Can you work these out from the model? Positions are in its coordinate system, mm. Face numbers are marked on the shaded views. A direction names the side the tool comes from. Give positions to 0.01 mm unless a question says otherwise; leave off trailing zeros. Order: outer loops, then holes, each group sorted by start corner. A loop starts at its lowest first (then second) coordinate and runs counter-clockwise, first axis right, second up. Notation, with made-up numbers: M 78.25,-22.75 L 135.25,-22.75 A21 cw 135.25,13.25 Z; hole C 5,-28.75 d1. An arc over 180 degrees is marked long. Use one line per item in the form item = value. Start each with the question number.
1. We'd pull the mould along Z, two halves only. Please class the marked faces 6, 7 and 8: +Z half, -Z half, draft (parallel to the pull), parting line (faces both ways), or undercut.
2. For the marked faces 1, 2, 3, 4 and 5, which set-ups out of +Z, -Z, +X, -X, +Y, -Y let a thin tool reach every point of the face, with its end or its side?
3. I want a section at D-D, the plane z = 0.5. List the corners of the cut face in (x, y) for me.
4. I want a section at C-C, the plane y = 12.5. List the corners of the cut face in (x, z) for me, and give its area (3 significant figures).
5. Will these pins go through, and if not, where does the flat tip stop? P1, Ø2.5, axis at x = -7, z = 0, coming from the -Y side; P2, Ø3, axis at y = 0.5, z = -7, coming from the -X side; P3, Ø8.5, axis at x = -4.5, y = -3, coming from the +Z side; P4, Ø1, axis at x = -8, z = -4.5, coming from the -Y side.
6. I want a section at B-B, the plane x = 5.5. List the corners of the cut face in (y, z) for me.
7. I want a section at A-A, the plane z = 4.5. List the corners of the cut face in (x, y) for me, and give its area (3 significant figures).
8. I need wall thicknesses on L1, parallel to X at y = 7, z = -5.25; L2, parallel to Z at x = 8.5, y = 3; L3, parallel to X at y = -10, z = -8. Which ranges of each line are inside material? Lowest first, please.
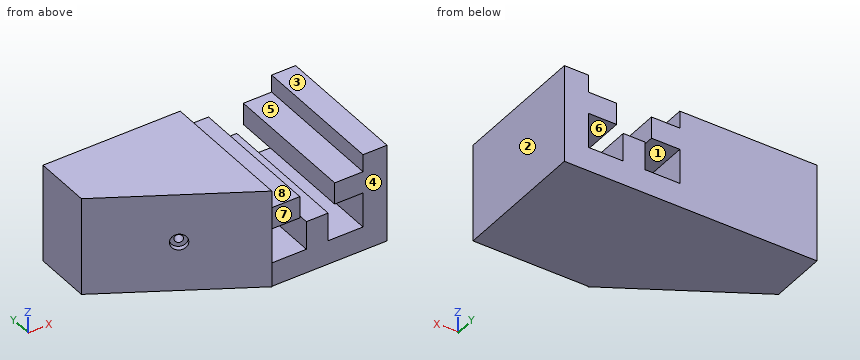
```python
from build123d import *

# Parameters (mm, degrees)
BOSS_EXTRU_1_DEPTH                               = 15
ESQUISSE1_W                                      = 21.65
ESQUISSE1_H                                      = 30
BOSS_EXTRU_2_DEPTH                               = 25
ESQUISSE3_W                                      = 30.3
ESQUISSE3_H                                      = 21.65
BOSS_EXTRU_3_DEPTH                               = 25
ENL_V_MAT_EXTRU_2_DEPTH                          = 61.834878976
ENL_V_MAT_EXTRU_2_DEPTH_BACK                     = 61.834878976
CHAMBRAGE_POUR_VIS_T_TE_RONDE_BOMB_E_D           = 1.778
CHAMBRAGE_POUR_VIS_T_TE_RONDE_BOMB_E_DEPTH       = 12
CHAMBRAGE_POUR_VIS_T_TE_RONDE_BOMB_E_CBORE_D     = 3.57124
CHAMBRAGE_POUR_VIS_T_TE_RONDE_BOMB_E_CBORE_DEPTH = 1.1176
CHAMBRAGE_POUR_VIS_T_TE_RONDE_BOMB_E_TIP         = 0.53416509


with BuildPart() as part:
    # Base → Boss.-Extru.1 (new, symmetric)
    with BuildSketch(Plane(origin=(0, 0, 0), x_dir=(1, 0, 0), z_dir=(0, 1, 0))):
        Polygon((-3.85, -2.4), (-3.85, 2.4), (-10.1, 2.4), (-10.1, 10.1), (-2.4, 10.1), (-2.4, 3.85), (2.4, 3.85), (2.4, 10.1), (10.1, 10.1), (10.1, 2.4), (3.85, 2.4), (3.85, -2.4), (10.1, -2.4), (10.1, -6.25), (15.4, -6.25), (15.4, 15.4), (-15.4, 15.4), (-15.4, -6.25), (-10.1, -6.25), (-10.1, -2.4), align=None)
    extrude(amount=BOSS_EXTRU_1_DEPTH, both=True)

    # Esquisse1 → Boss.-Extru.2 (add)
    with BuildSketch(Plane.ZY.offset(15.4)):
        with Locations((-4.575, 0)):
            Rectangle(ESQUISSE1_W, ESQUISSE1_H)
    extrude(amount=BOSS_EXTRU_2_DEPTH)

    # Esquisse3 → Boss.-Extru.3 (add)
    with BuildSketch(Plane.XZ.offset(15)):
        with Locations((-25.25, -4.575)):
            Rectangle(ESQUISSE3_W, ESQUISSE3_H)
    extrude(amount=BOSS_EXTRU_3_DEPTH)

    # Esquisse4 → Enlèv. mat.-Extru.2 (cut, two sides: drawn at the far end of the back side and taken through both)
    with BuildSketch(Plane.XY.offset(6.25).offset(-ENL_V_MAT_EXTRU_2_DEPTH_BACK)):
        Polygon((119.921926151, -90.183707408), (-10.1, -15.115513344), (-40.4, 2.378199813), (-170.421926151, 77.446393876), (-320.558314278, -182.597458425), (-30.214461977, -350.227559709), align=None)
    extrude(amount=ENL_V_MAT_EXTRU_2_DEPTH + ENL_V_MAT_EXTRU_2_DEPTH_BACK, mode=Mode.SUBTRACT)

    # Chambrage pour vis à tête ronde bombée #02
    with Locations(Plane(origin=(-9.070209274, -15.710063297, 0), x_dir=(-0.8660254037844364, 0.5000000000000041, 0), z_dir=(-0.500000000000004, -0.8660254037844363, 0))):
        with Locations((18.233273003, 4.443374623)):
            CounterBoreHole(CHAMBRAGE_POUR_VIS_T_TE_RONDE_BOMB_E_D / 2, CHAMBRAGE_POUR_VIS_T_TE_RONDE_BOMB_E_CBORE_D / 2, CHAMBRAGE_POUR_VIS_T_TE_RONDE_BOMB_E_CBORE_DEPTH, depth=CHAMBRAGE_POUR_VIS_T_TE_RONDE_BOMB_E_DEPTH)
            with Locations((0, 0, -(CHAMBRAGE_POUR_VIS_T_TE_RONDE_BOMB_E_DEPTH + CHAMBRAGE_POUR_VIS_T_TE_RONDE_BOMB_E_TIP / 2))):  # 118° drill point
                Cone(0, CHAMBRAGE_POUR_VIS_T_TE_RONDE_BOMB_E_D / 2, CHAMBRAGE_POUR_VIS_T_TE_RONDE_BOMB_E_TIP, mode=Mode.SUBTRACT)


solid = part.part
```
Check result:
q1.face_6 = undercut
q1.face_7 = draft
q1.face_8 = +Z half
q2.face_1 = +Y, -Y
q2.face_2 = +Z, -Z, +X, +Y, -Y
q2.face_3 = +Z, +X, -X, +Y, -Y
q2.face_4 = +Z, -Z, +X, -Y
q2.face_5 = +Z, +Y, -Y
q3.outline = M -40.4,2.38 L -10.1,-15.12 L -10.1,-15 L -3.85,-15 L -3.85,15 L -40.4,15 Z; M 3.85,-15 L 15.4,-15 L 15.4,15 L 3.85,15 Z
q4.outline = M -40.4,-15.4 L 15.4,-15.4 L 15.4,6.25 L 10.1,6.25 L 10.1,2.4 L 3.85,2.4 L 3.85,-2.4 L 10.1,-2.4 L 10.1,-10.1 L 2.4,-10.1 L 2.4,-3.85 L -2.4,-3.85 L -2.4,-10.1 L -10.1,-10.1 L -10.1,-2.4 L -3.85,-2.4 L -3.85,2.4 L -10.1,2.4 L -10.1,6.25 L -40.4,6.25 Z
q4.area = 968 mm2
q5.P1 = -15
q5.P2 = -39.74
q5.P3 = 2.4
q5.P4 = through
q6.outline = M -15,-15.4 L 15,-15.4 L 15,-10.1 L -15,-10.1 Z; M -15,-2.4 L 15,-2.4 L 15,2.4 L -15,2.4 Z
q7.outline = M -40.4,2.38 L -10.1,-15.12 L -10.1,15 L -40.4,15 Z; M 10.1,-15 L 15.4,-15 L 15.4,15 L 10.1,15 Z
q7.area = 806 mm2
q8.L1 = -40.4 to -10.1, -2.4 to 2.4, 10.1 to 15.4
q8.L2 = -15.4 to -10.1, -2.4 to 2.4
q8.L3 = -18.96 to -10.1, -2.4 to 2.4, 10.1 to 15.4
